```python
from build123d import *

# Parameters (mm, degrees)
SKETCH1_W           = 45.5
SKETCH1_H           = 32
BOSS_EXTRUDE1_DEPTH = 10
SKETCH2_W           = 40.7
SKETCH2_H           = 27.02
CUT_EXTRUDE1_DEPTH  = 8
SKETCH3_W           = 32
SKETCH3_H           = 10
BOSS_EXTRUDE2_DEPTH = 5.6
SKETCH4_W           = 3
SKETCH4_H           = 32
BOSS_EXTRUDE3_DEPTH = 20


with BuildPart() as part:
    # Sketch1 → Boss-Extrude1 (new body)
    with BuildSketch(Plane(origin=(0, 0, 0), x_dir=(1, 0, 0), z_dir=(0, 1, 0))):
        with Locations((22.75, 16)):
            Rectangle(SKETCH1_W, SKETCH1_H)
    extrude(amount=BOSS_EXTRUDE1_DEPTH)

    # Sketch2 → Cut-Extrude1 (cut)
    with BuildSketch(Plane(origin=(0, 10, 0), x_dir=(1, 0, 0), z_dir=(0, 1, 0))):
        with Locations((22.749993038, 16.000024748)):
            Rectangle(SKETCH2_W, SKETCH2_H)
    extrude(amount=-CUT_EXTRUDE1_DEPTH, mode=Mode.SUBTRACT)

    # Sketch3 → Boss-Extrude2 (add)
    with BuildSketch(Plane.ZY):
        with Locations((-16, 5)):
            Rectangle(SKETCH3_W, SKETCH3_H)
    extrude(amount=BOSS_EXTRUDE2_DEPTH)

    # Sketch4 → Boss-Extrude3 (add)
    with BuildSketch(Plane(origin=(0, 10, 0), x_dir=(1, 0, 0), z_dir=(0, 1, 0))):
        with Locations((-4.1, 16)):
            Rectangle(SKETCH4_W, SKETCH4_H)
    extrude(amount=BOSS_EXTRUDE3_DEPTH)


solid = part.part
```
Can you work these out from the model? Positions are in its coordinate system, mm. A direction names the side the tool comes from. Give positions to 0.01 mm unless a question says otherwise; leave off trailing zeros. Loops run counter-clockwise (first coordinate to the right, second up) from the corner with the lowest first, then second, coordinate; pieces in that order, holes last. Notation, with made-up numbers: M -17,50.25 L 2,50.25 A8 ccw 2,63.25 Z; hole C -22.75,55.25 d2. An arc over 180 degrees is marked long. Use CSV: the item, a comma, the result in double quotes. Start each with the question number.
1. On a 3-axis mill with a long thin cutter (end or side, diameter ignored), from which of +Z, -Z, +X, -X, +Y, -Y can I reach the whole of each face in a straight line? I mean faces 1 (the face through (14, 8, 0)), 2 (the face through (-2.6, 20, -16)), 3 (the face through (22, 6, -29.51)). Say none if no direction works.
2. Imagine slicing it at C-C, the plane x = 41.5. Write out the boundary of the cut face in (y, z).
3. Imagine slicing it at B-B, the plane z = -6.5. Write out the boundary of the cut face in (x, y).
4. For P1, Ø8, axis at x = 23, z = -23.5, coming from the +Y side, with a flat end and sliding along its axis, tell me the tip position at first contact or that it passes through.
5. If I drill on L1, parallel to X at y = 8, z = -10.5; L2, parallel to Z at x = 8.5, y = 5.25; L3, parallel to Y at x = 3, z = -8.5, over which ranges is the centre line in solid material (lowest first)?
6. If we mould it in two halves opening along Z, with no side actions, what happens to faces 4 (the face through (22, 10, -2)), 5 (the face through (2.4, 6, -16)), 6 (the face through (14, 8, -32)), 7 (the face through (22, 2, -16))? For each: released by +Z, released by -Z, zero draft, split by the parting line, or undercut.
7. Imagine slicing it at A-A, the plane y = 4.75. Write out the boundary of the cut face in (x, z).
8. Imagine slicing it at D-D, the plane y = 12. Write out the boundary of the cut face in (x, z), plus the area to 3 significant figures.
Response values:
1,face 1,"+Z, +X, -X, +Y, -Y"
1,face 2,"+Z, -Z, +X, +Y"
1,face 3,"+Y"
2,outline,"M 0,-32 L 10,-32 L 10,-29.51 L 2,-29.51 L 2,-2.49 L 10,-2.49 L 10,0 L 0,0 Z"
3,outline,"M -5.6,0 L 45.5,0 L 45.5,10 L 43.1,10 L 43.1,2 L 2.4,2 L 2.4,10 L -2.6,10 L -2.6,30 L -5.6,30 Z"
4,P1,"y = 2"
5,L1,"-5.6 to 2.4, 43.1 to 45.5"
5,L2,"-32 to -29.51, -2.49 to 0"
5,L3,"0 to 2"
6,face 4,"zero draft"
6,face 5,"undercut"
6,face 6,"released by -Z"
6,face 7,"undercut"
7,outline,"M -5.6,-32 L 45.5,-32 L 45.5,0 L -5.6,0 Z; hole M 2.4,-29.51 L 43.1,-29.51 L 43.1,-2.49 L 2.4,-2.49 Z"
8,outline,"M -5.6,-32 L -2.6,-32 L -2.6,0 L -5.6,0 Z"
8,area,"96.0 mm^2"
